```python
from build123d import *

# Parameters (mm, degrees)
REVOLVE1_ANGLE                 = 90.0000000000002
BOSS_EXTRUDE2_DEPTH            = 22.5
CUT_EXTRUDE1_DEPTH             = 41.736973886583954
MIRROR3_START                  = -2.736132077
MIRROR3_DEPTH                  = 5
MIRROR3_START_2                = 2.263867923
MIRROR3_2_DEPTH                = 20.236132077
MIRROR3_3_DEPTH                = 1
MIRROR3_START_3                = 1.263867923
MIRROR3_4_DEPTH                = 1
MIRROR4_START                  = -2.736132077
MIRROR4_DEPTH                  = 5
MIRROR4_START_2                = 2.263867923
MIRROR4_2_DEPTH                = 20.236132077
MIRROR4_3_DEPTH                = 1
MIRROR4_START_3                = 1.263867923
MIRROR4_4_DEPTH                = 1
SKETCH7_R                      = 3.35
CUT_EXTRUDE2_DEPTH             = 20
FILLET9_R                      = 0.5
CUT_EXTRUDE3_REACH             = 43.908
SKETCH8_R                      = 1.5000000000000004
CUT_EXTRUDE3_DIRECTION_2_REACH = 43.908


# Read off the part's stored shape, not the designer's step: Mirror3, Mirror4
with BuildPart() as part:
    # Sketch1 → Revolve1 (revolve)
    with BuildSketch(Plane.XY):
        Polygon((0, 2.2638679230386933), (0, -2.7361320769613027), (25, -2.7361320769613027), (25.000000000000007, -1.736132076961303), (24.750000000000007, -1.736132076961303), (24.75, 1.2638679230386973), (25, 1.2638679230386973), (25, 2.2638679230386973), align=None)
    revolve(axis=Axis((0, 2.2638679230386933, 0), (0, -1, 0)), revolution_arc=REVOLVE1_ANGLE)

    # Sketch2 → Boss-Extrude2 (add)
    with BuildSketch(Plane(origin=(0, 0, 0), x_dir=(1, 0, 0), z_dir=(0, 1, 0))):
        with BuildLine():
            Line((0, 0), (6, 0))
            ThreePointArc((6, 0), (4.242640687119239, -4.242640687119332), (-1.3093e-13, -6))
            Line((-1.3093e-13, -6), (0, 0))
        make_face()
    extrude(amount=BOSS_EXTRUDE2_DEPTH)

    # Sketch6 → Cut-Extrude1 (cut, through all)
    with BuildSketch(Plane(origin=(0, 2.263867923038695, 0), x_dir=(1, 0, 0), z_dir=(0, 1, 0))):
        with BuildLine():
            Line((1.4999999999999127, -5.809475019311148), (1.4999999999999145, -20.946360065653423))
            ThreePointArc((1.4999999999999145, -20.946360065653423), (14.849242404917469, -14.849242404917533), (20.946360065653415, -1.5))
            Line((20.946360065653415, -1.5), (5.809475019311125, -1.5))
            ThreePointArc((5.809475019311125, -1.5), (4.242640687119254, -4.242640687119317), (1.4999999999999127, -5.809475019311148))
        make_face()
    extrude(amount=-CUT_EXTRUDE1_DEPTH, mode=Mode.SUBTRACT)

    # Mirror3 outline → Mirror3 (add)
    with BuildSketch(Plane(origin=(0, 0, 0), x_dir=(1, 0, 0), z_dir=(0, 1, 0)).offset(MIRROR3_START)):
        with BuildLine():
            ThreePointArc((24.75, 0), (17.500892834, 17.500892834), (0, 24.75))
            Line((0, 24.75), (0, 0))
            Line((0, 0), (24.75, 0))
        make_face()
        with BuildLine():
            Line((20.946360066, 1.5), (5.809475019, 1.5))
            ThreePointArc((5.809475019, 1.5), (4.242640687, 4.242640687), (1.5, 5.809475019))
            Line((1.5, 5.809475019), (1.5, 20.946360066))
            ThreePointArc((1.5, 20.946360066), (14.849242405, 14.849242405), (20.946360066, 1.5))
        make_face(mode=Mode.SUBTRACT)
    extrude(amount=MIRROR3_DEPTH)

    # Mirror3 2 outline → Mirror3 2 (add)
    with BuildSketch(Plane(origin=(0, 0, 0), x_dir=(1, 0, 0), z_dir=(0, 1, 0)).offset(MIRROR3_START_2)):
        with BuildLine():
            Line((0, 0), (6, 0))
            ThreePointArc((6, 0), (4.242640687, 4.242640687), (0, 6))
            Line((0, 6), (0, 0))
        make_face()
    extrude(amount=MIRROR3_2_DEPTH)

    # Mirror3 3 outline → Mirror3 3 (add)
    with BuildSketch(Plane(origin=(0, 0, 0), x_dir=(1, 0, 0), z_dir=(0, 1, 0)).offset(MIRROR3_START)):
        with BuildLine():
            Line((24.75, 0), (25, 0))
            ThreePointArc((25, 0), (17.67766953, 17.67766953), (0, 25))
            Line((0, 25), (0, 24.75))
            ThreePointArc((0, 24.75), (17.500892834, 17.500892834), (24.75, 0))
        make_face()
    extrude(amount=MIRROR3_3_DEPTH)

    # Mirror3 4 outline → Mirror3 4 (add)
    with BuildSketch(Plane(origin=(0, 0, 0), x_dir=(1, 0, 0), z_dir=(0, 1, 0)).offset(MIRROR3_START_3)):
        with BuildLine():
            Line((24.75, 0), (25, 0))
            ThreePointArc((25, 0), (17.67766953, 17.67766953), (0, 25))
            Line((0, 25), (0, 24.75))
            ThreePointArc((0, 24.75), (17.500892834, 17.500892834), (24.75, 0))
        make_face()
    extrude(amount=MIRROR3_4_DEPTH)

    # Mirror4 outline → Mirror4 (add)
    with BuildSketch(Plane(origin=(0, 0, 0), x_dir=(1, 0, 0), z_dir=(0, 1, 0)).offset(MIRROR4_START)):
        with BuildLine():
            ThreePointArc((0, 24.75), (-24.75, 0), (0, -24.75))
            Line((0, -24.75), (0, 24.75))
        make_face()
        with BuildLine():
            Line((-1.5, 20.946360066), (-1.5, 5.809475019))
            ThreePointArc((-1.5, 5.809475019), (-4.242640687, 4.242640687), (-5.809475019, 1.5))
            Line((-5.809475019, 1.5), (-20.946360066, 1.5))
            ThreePointArc((-20.946360066, 1.5), (-14.849242405, 14.849242405), (-1.5, 20.946360066))
        make_face(mode=Mode.SUBTRACT)
        with BuildLine():
            Line((-20.946360066, -1.5), (-5.809475019, -1.5))
            ThreePointArc((-5.809475019, -1.5), (-4.242640687, -4.242640687), (-1.5, -5.809475019))
            Line((-1.5, -5.809475019), (-1.5, -20.946360066))
            ThreePointArc((-1.5, -20.946360066), (-14.849242405, -14.849242405), (-20.946360066, -1.5))
        make_face(mode=Mode.SUBTRACT)
    extrude(amount=MIRROR4_DEPTH)

    # Mirror4 2 outline → Mirror4 2 (add)
    with BuildSketch(Plane(origin=(0, 0, 0), x_dir=(1, 0, 0), z_dir=(0, 1, 0)).offset(MIRROR4_START_2)):
        with BuildLine():
            Line((0, -6), (0, 6))
            ThreePointArc((0, 6), (-6, 0), (0, -6))
        make_face()
    extrude(amount=MIRROR4_2_DEPTH)

    # Mirror4 3 outline → Mirror4 3 (add)
    with BuildSketch(Plane(origin=(0, 0, 0), x_dir=(1, 0, 0), z_dir=(0, 1, 0)).offset(MIRROR4_START)):
        with BuildLine():
            Line((0, 24.75), (0, 25))
            ThreePointArc((0, 25), (-25, 0), (0, -25))
            Line((0, -25), (0, -24.75))
            ThreePointArc((0, -24.75), (-24.75, 0), (0, 24.75))
        make_face()
    extrude(amount=MIRROR4_3_DEPTH)

    # Mirror4 4 outline → Mirror4 4 (add)
    with BuildSketch(Plane(origin=(0, 0, 0), x_dir=(1, 0, 0), z_dir=(0, 1, 0)).offset(MIRROR4_START_3)):
        with BuildLine():
            Line((0, 24.75), (0, 25))
            ThreePointArc((0, 25), (-25, 0), (0, -25))
            Line((0, -25), (0, -24.75))
            ThreePointArc((0, -24.75), (-24.75, 0), (0, 24.75))
        make_face()
    extrude(amount=MIRROR4_4_DEPTH)

    # Sketch7 → Cut-Extrude2 (cut)
    with BuildSketch(Plane(origin=(0, 22.5, 0), x_dir=(1, 0, 0), z_dir=(0, 1, 0))):
        with Locations(Location((0, 0, 0), (0, 0, 270))):
            Circle(SKETCH7_R)
    extrude(amount=-CUT_EXTRUDE2_DEPTH, mode=Mode.SUBTRACT)

    # Fillet9
    # the kernel refuses this fillet: 0.5 mm, written as the material it adds along each edge
    with BuildSketch(Plane(origin=(3.55e-15, 1.263867923, 0), x_dir=(-1.4e-16, 0, 1), z_dir=(1, 0, 1.4e-16))) as fillet9_piece_1:
        with BuildLine():
            CenterArc((25.25, 0.4330127018922456), FILLET9_R, 180, 60.000000000001876)
            Line((25.000000000000014, 1.821e-14), (24.995000000000015, -0.00866025403782644))
            ThreePointArc((24.995000000000015, -0.00866025403782644), (24.875000000000007, -0.01000000000000001), (24.75, -0.01000000000000001))
            Line((24.75, -0.01000000000000001), (24.74, 0))
            Line((24.74, 0), (24.74, 0.4330127018922456))
            Line((24.74, 0.4330127018922456), (24.75, 0.4330127018922456))
        make_face()
    revolve(axis=Axis((3.55e-15, 1.263867923, 0), (0, -1, 0)), revolution_arc=179.99999999999997)
    with BuildSketch(Plane(origin=(3.55e-15, -1.7361320770000002, 0), x_dir=(-1.4e-16, 0, 1), z_dir=(1, 0, 1.4e-16))) as fillet9_piece_2:
        with BuildLine():
            CenterArc((25.25, -0.4330127018922456), FILLET9_R, 119.99999999999814, 60.00000000000186)
            Line((24.75, -0.4330127018922456), (24.74, -0.4330127018922456))
            Line((24.74, -0.4330127018922456), (24.74, 0))
            Line((24.74, 0), (24.75, 0.01000000000000001))
            ThreePointArc((24.75, 0.01000000000000001), (24.875000000000007, 0.01000000000000001), (24.995000000000015, 0.00866025403782644))
            Line((24.995000000000015, 0.00866025403782644), (25.000000000000014, -1.821e-14))
        make_face()
    revolve(axis=Axis((3.55e-15, -1.7361320770000002, 0), (0, -1, 0)), revolution_arc=179.99999999999997)
    with BuildSketch(Plane(origin=(0, -1.7361320769613031, 0), x_dir=(1, 0, 0), z_dir=(0, 0, -1))) as fillet9_piece_3:
        with BuildLine():
            CenterArc((25.250000000000007, -0.4330127018922436), FILLET9_R, 119.9999999999986, 60.00000000000141)
            Line((24.750000000000007, -0.4330127018922436), (24.740000000000006, -0.4330127018922436))
            Line((24.740000000000006, -0.4330127018922436), (24.740000000000006, 0))
            Line((24.740000000000006, 0), (24.750000000000007, 0.01000000000000001))
            ThreePointArc((24.750000000000007, 0.01000000000000001), (24.875000000000014, 0.01000000000000001), (24.99500000000002, 0.00866025403782622))
            Line((24.99500000000002, 0.00866025403782622), (25.000000000000018, -1.821e-14))
        make_face()
    revolve(axis=Axis((0, -1.7361320769613031, 0), (0, -1, 0)), revolution_arc=90.0000000000002)
    with BuildSketch(Plane(origin=(-1.25320021e-09, -1.7361320770000002, 1.25320021e-09), x_dir=(5.063435192760357e-11, 0, -1.0), z_dir=(-1.0, 0, -5.063435192760357e-11))) as fillet9_piece_4:
        with BuildLine():
            CenterArc((25.2500000012532, -0.4330127018922456), FILLET9_R, 119.99999999999814, 60.00000000000186)
            Line((24.7500000012532, -0.4330127018922456), (24.7400000012532, -0.4330127018922456))
            Line((24.7400000012532, -0.4330127018922456), (24.7400000012532, 0))
            Line((24.7400000012532, 0), (24.7500000012532, 0.01000000000000001))
            ThreePointArc((24.7500000012532, 0.01000000000000001), (24.875000001253206, 0.01000000000000001), (24.995000001253217, 0.00866025403782644))
            Line((24.995000001253217, 0.00866025403782644), (25.000000001253213, -1.821e-14))
        make_face()
    revolve(axis=Axis((-1.25320021e-09, -1.7361320770000002, 1.25320021e-09), (0, -1, 0)), revolution_arc=89.99999999419774)
    with BuildSketch(Plane(origin=(0, 1.2638679230386973, 0), x_dir=(1, 0, 0), z_dir=(0, 0, -1))) as fillet9_piece_5:
        with BuildLine():
            CenterArc((25.250000000000007, 0.4330127018922396), FILLET9_R, 180, 60.000000000000455)
            Line((25.00000000000001, 1.821e-14), (24.99500000000001, -0.00866025403782622))
            ThreePointArc((24.99500000000001, -0.00866025403782622), (24.875000000000007, -0.01000000000000001), (24.75, -0.01000000000000001))
            Line((24.75, -0.01000000000000001), (24.74, 0))
            Line((24.74, 0), (24.740000000000006, 0.4330127018922396))
            Line((24.740000000000006, 0.4330127018922396), (24.750000000000007, 0.4330127018922396))
        make_face()
    revolve(axis=Axis((0, 1.2638679230386973, 0), (0, -1, 0)), revolution_arc=90.0000000000002)
    with BuildSketch(Plane(origin=(-1.25320021e-09, 1.263867923, 1.25320021e-09), x_dir=(5.063435192760357e-11, 0, -1.0), z_dir=(-1.0, 0, -5.063435192760357e-11))) as fillet9_piece_6:
        with BuildLine():
            CenterArc((25.2500000012532, 0.4330127018922456), FILLET9_R, 180, 60.000000000001876)
            Line((25.000000001253213, 1.821e-14), (24.995000001253217, -0.00866025403782644))
            ThreePointArc((24.995000001253217, -0.00866025403782644), (24.875000001253206, -0.01000000000000001), (24.7500000012532, -0.01000000000000001))
            Line((24.7500000012532, -0.01000000000000001), (24.7400000012532, 0))
            Line((24.7400000012532, 0), (24.7400000012532, 0.4330127018922456))
            Line((24.7400000012532, 0.4330127018922456), (24.7500000012532, 0.4330127018922456))
        make_face()
    revolve(axis=Axis((-1.25320021e-09, 1.263867923, 1.25320021e-09), (0, -1, 0)), revolution_arc=89.99999999419774)

    # Sketch8 → Cut-Extrude3 (cut, up to next)
    with BuildSketch(Plane.XY, mode=Mode.PRIVATE) as cut_extrude3_sk1:
        with Locations(Location((1.22e-15, 12.499999999999998, 0), (0, 0, 180))):
            Circle(SKETCH8_R)
    cut_extrude3_tool1 = extrude(cut_extrude3_sk1.sketch, amount=CUT_EXTRUDE3_REACH, mode=Mode.PRIVATE) & part.part
    add(cut_extrude3_tool1.solids().sort_by_distance((0, 12.5, 0))[0], mode=Mode.SUBTRACT)

    # Sketch8 → Cut-Extrude3 direction 2 (cut, up to next)
    with BuildSketch(Plane.XY, mode=Mode.PRIVATE) as cut_extrude3_direction_2_sk1:
        with Locations(Location((1.22e-15, 12.499999999999998, 0), (0, 0, 180))):
            Circle(SKETCH8_R)
    cut_extrude3_direction_2_tool1 = extrude(cut_extrude3_direction_2_sk1.sketch, amount=-CUT_EXTRUDE3_DIRECTION_2_REACH, mode=Mode.PRIVATE) & part.part
    add(cut_extrude3_direction_2_tool1.solids().sort_by_distance((0, 12.5, 0))[0], mode=Mode.SUBTRACT)


solid = part.part
```
Can you work these out from the model? Positions are in its coordinate system, mm. A direction names the side the tool comes from. Round coordinates to 2 decimals unless told otherwise and drop trailing zeros. Order: outer loops, then holes, each group sorted by start corner. A loop starts at its lowest first (then second) coordinate and runs counter-clockwise, first axis right, second up.
(1) If we section it at A-A (y = 12.5): Please give me the cut outline in (x, z).
Results are:
outline: (-1.5, -5.81) - (-1.5, -3) arc R3.35 cw to (-1.5, 3) - (-1.5, 5.81) arc R6 ccw to start; (1.5, -5.81) arc R6 ccw to (1.5, 5.81) - (1.5, 3) arc R3.35 cw to (1.5, -3) - close
(2) On a 3-axis mill with a long thin cutter (end or side, diameter ignored), from which of +Z, -Z, +X, -X, +Y, -Y can I reach the whole of each face in a straight line? I mean faces 1 (the face through (0, 2.5, 0)), 2 (the face through (-13, 0, -1.5)), 3 (the face through (-1.386, 13.075, -4.477)). Say none if no direction works.
Results are:
face 1: +Y
face 2: +Y, -Y
face 3: +Z, -Z
(3) If we section it at B-B (x = 18): Count the separate pieces of the cut face and the enclosed holes in it, plus the area to 3 significant figures.
Results are:
separate pieces: 3
enclosed holes: 0
area: 78.3 mm2
(4) We'd pull the mould along Z, two halves only. Please class faces 4 (the face through (13, 0, 1.5)), 5 (the face through (-1.386, 13.075, 4.477)): +Z half, -Z half, draft (parallel to the pull), parting line (faces both ways), or undercut.
Results are:
face 4: undercut
face 5: draft
(5) If I drill on L1, parallel to X at y = 2, z = -9.5; L2, parallel to X at y = 2, z = 14.5; L3, parallel to Y at x = 0, z = 4, over which ranges is the centre line in solid material (lowest first)?
Results are:
L1: x = -23.12 to -18.73, -1.5 to 1.5, 18.73 to 23.12
L2: x = -20.37 to -15.19, -1.5 to 1.5, 15.19 to 20.37
L3: y = -2.74 to 11, 14 to 22.5
(6) I'm going to push flat-ended pins straight in: pin 1 (5.5 mm diameter, centred on x = -14.5, y = 0.5, fed in from -Z); pin 2 (5.5 mm diameter, centred on y = -0.5, z = 13, fed in from -X); pin 3 (6 mm diameter, centred on x = 6.5, y = 16.5, fed in from +Z). Where does each tip first touch, or does it pass through?
Results are:
pin 1: stops at z = -22.01
pin 2: stops at x = -22.67
pin 3: stops at z = 4.87
(7) If we section it at D-D (y = 6.5): Please give me the cut outline in (x, z), plus the area to 3 significant figures.
Results are:
outline: circle Ø12 at (0, 0); hole circle Ø6.7 at (0, 0)
area: 77.8 mm2
